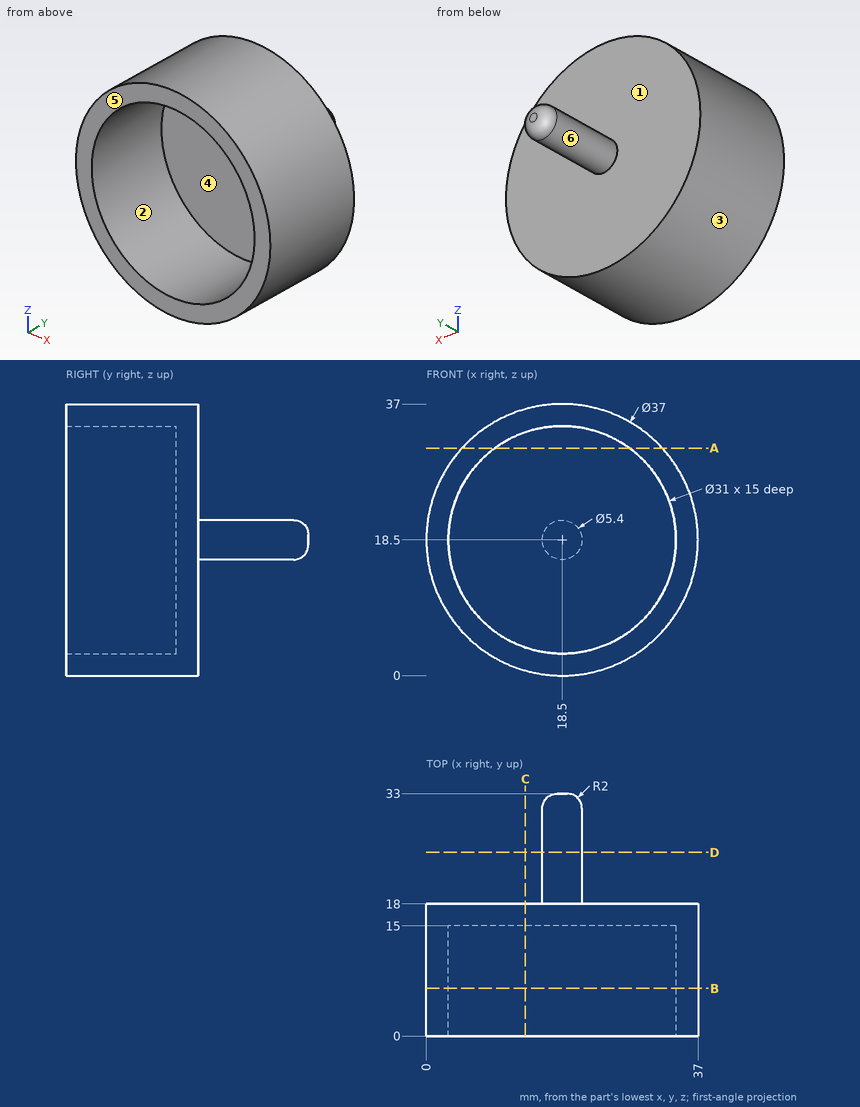
Drawing for the job (mm, zero at the part's lowest x, y, z). A direction names the side the tool comes from. Give positions to 0.01 mm unless a question says otherwise; leave off trailing zeros. Write each loop counter-clockwise with the first axis right and the second up, starting at its lowest first coordinate (ties: lowest second). Pieces come first, ordered by that corner, then holes. Notation, with made-up numbers: M -23,-20.75 L 22,-20.75 A19 cw 22,10.25 Z; hole C -8.5,45 d4. An arc over 180 degrees is marked long. Use CSV: the item, a comma, the result in double quotes.
Item 1: Drill centre lines: probe 1 along Z at (x, y) = (18, 10); probe 2 along Y at (x, z) = (25.5, 22). Where is each one in solid material? Low to high.
Taken from the geometry:
probe 1,"z = 0.01 to 3.01, 33.99 to 36.99"
probe 2,"y = 15 to 18"
Item 2: Slice it at D-D on y = 25. Write the cut outline in (x, z), plus the area to 3 significant figures.
Taken from the geometry:
outline,"C 18.5,18.5 d5.4"
area,"22.9 mm²"
Item 3: Slice it at A-A on z = 31. Write the cut outline in (x, y).
Taken from the geometry:
outline,"M 4.86,0 L 9.33,0 L 9.33,15 L 27.67,15 L 27.67,0 L 32.14,0 L 32.14,18 L 4.86,18 Z"
Item 4: Slice it at B-B on y = 6.5. Write the cut outline in (x, z).
Taken from the geometry:
outline,"C 18.5,18.5 d37; hole C 18.5,18.5 d31"
Item 5: Pull direction X, two halves, no side cores. Call the marked faces 1, 2 and 3: +X half, -X half, draft (parallel to the pull), parting line (faces both ways), or undercut.
Taken from the geometry:
face 1,"draft"
face 2,"undercut"
face 3,"parting line"
Item 6: Slice it at C-C on x = 13.5. Write the cut outline in (y, z), plus the area to 3 significant figures.
Taken from the geometry:
outline,"M 0,0.69 L 18,0.69 L 18,36.31 L 0,36.31 L 0,33.17 L 15,33.17 L 15,3.83 L 0,3.83 Z"
area,"201 mm²"
Item 7: Pin check, flat tips, straight feed: P1, Ø3, axis at y = 19, z = 8, coming from the +X side; P2, Ø1, axis at x = 3.5, z = 28, coming from the +Y side; P3, Ø1, axis at y = 6.5, z = 22.5, coming from the -X side. Stop position of each tip, or through.
Taken from the geometry:
P1,"stops at x = 34.44"
P2,"stops at y = 18"
P3,"stops at x = 0.33"
Item 8: Which spindle directions (+Z, -Z, +X, -X, +Y, -Y) get a long thin tool onto all of the face, cutting with end or side? Do the marked faces 4, 5 and 6. Say none if no direction does.
Taken from the geometry:
face 4,"-Y"
face 5,"+Z, -Z, +X, -X, -Y"
face 6,"+Y"
